Can you work these out from the drawing? Everything is in mm from the part's minimum corner. Round coordinates to 2 decimals unless told otherwise and drop trailing zeros. Loops run counter-clockwise (first coordinate to the right, second up) from the corner with the lowest first, then second, coordinate; pieces in that order, holes last. Notation, with made-up numbers: (23, 10) - (57, 10) arc R23 ccw to (57, 19) - close; hole circle Ø3 at (50, 44). An arc over 180 degrees is marked (long way). Answer as a JSON object with one key per item and string values. Group by question number.
1) Will this pin go through, and if not, where does the flat tip stop? P1, Ø6, axis at x = 130, y = 9, coming from the -Z side.
2) If I drill on line 1 along X through (y, z) = (1, 38.5); line 2 along X through (y, z) = (10.75, 38); line 3 along Z through (x, y) = (38.1, 5), over which ranges is the centre line in solid material (lowest first)? Write a range as [from, to].
3) I want a section at A-A, the plane x = 114.3. Please give me the cut outline in (y, z).
4) I want a section at B-B, the plane z = 38.1. Please give me the cut outline in (x, y), then the cut area to 3 significant figures.
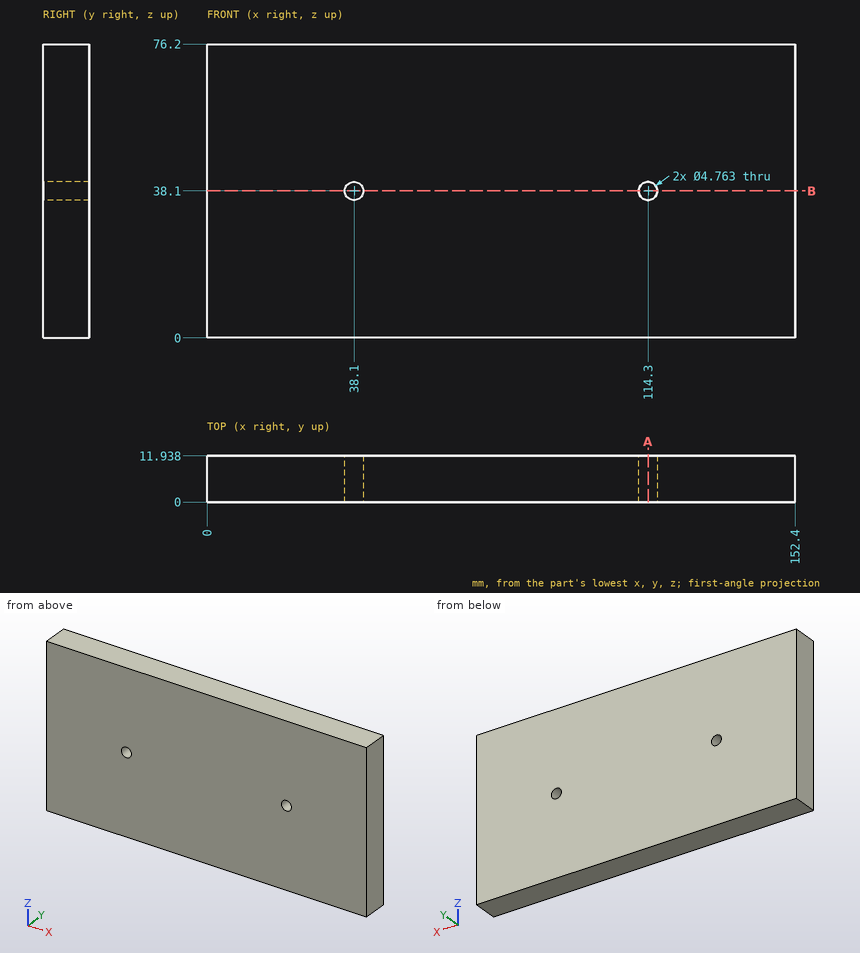
Outcome:
{
 "1": {"P1": "z = 0"},
 "2": {"line 1": "[0, 35.75], [40.45, 111.95], [116.65, 152.4]", "line 2": "[0, 35.72], [40.48, 111.92], [116.68, 152.4]", "line 3": "[0, 35.72], [40.48, 76.2]"},
 "3": {"outline": "(0, 0) - (11.94, 0) - (11.94, 35.72) - (0, 35.72) - close; (0, 40.48) - (11.94, 40.48) - (11.94, 76.2) - (0, 76.2) - close"},
 "4": {"outline": "(0, 0) - (35.72, 0) - (35.72, 11.94) - (0, 11.94) - close; (40.48, 0) - (111.92, 0) - (111.92, 11.94) - (40.48, 11.94) - close; (116.68, 0) - (152.4, 0) - (152.4, 11.94) - (116.68, 11.94) - close", "area": "1,710 mm^2"}
}
